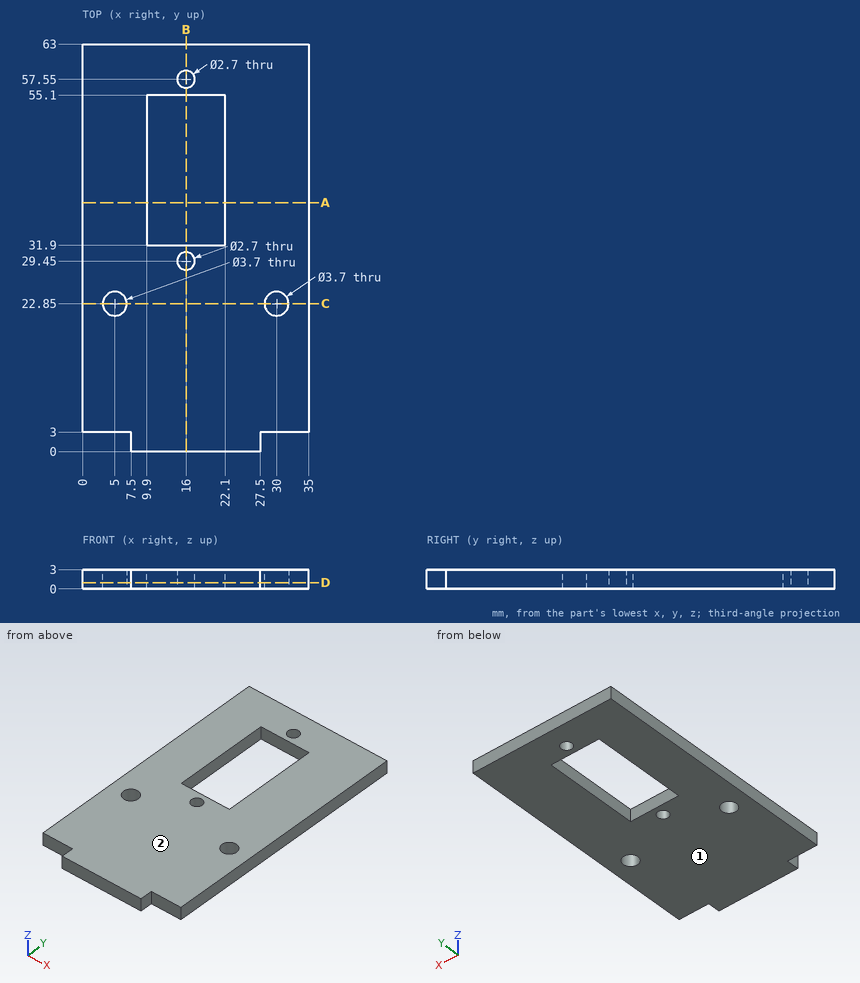
Here's the drawing with two shaded views (mm, measured from the low corner). I have some questions. Give positions to 0.01 mm unless a question says otherwise; leave off trailing zeros. Loops run counter-clockwise (first coordinate to the right, second up) from the corner with the lowest first, then second, coordinate; pieces in that order, holes last. Notation, with made-up numbers: M 14.25,0 L 35.25,0 A12 ccw 35.25,9 Z; hole C 5.5,40.25 d10. An arc over 180 degrees is marked long. One line per item, written item: value.
(1) Will these pins go through, and if not, where does the flat tip stop? pin 1 (0.9 mm diameter, centred on x = 5.5, z = 2, fed in from -Y); pin 2 (2 mm diameter, centred on x = 30, y = 22.85, fed in from +Z); pin 3 (5 mm diameter, centred on x = 5, y = 22.85, fed in from -Z).
Returned:
pin 1: y = 3
pin 2: through
pin 3: z = 0
(2) Suppose I cut it at D-D on z = 1. List the corners of the cut face in (x, y) for me.
Returned:
outline: M 0,3 L 7.5,3 L 7.5,0 L 27.5,0 L 27.5,3 L 35,3 L 35,63 L 0,63 Z; hole C 5,22.85 d3.7; hole M 9.9,31.9 L 22.1,31.9 L 22.1,55.1 L 9.9,55.1 Z; hole C 16,29.45 d2.7; hole C 16,57.55 d2.7; hole C 30,22.85 d3.7
(3) Suppose I cut it at C-C on y = 22.85. List the corners of the cut face in (x, z) for me.
Returned:
outline: M 0,0 L 3.15,0 L 3.15,3 L 0,3 Z; M 6.85,0 L 28.15,0 L 28.15,3 L 6.85,3 Z; M 31.85,0 L 35,0 L 35,3 L 31.85,3 Z
(4) I need wall thicknesses on line 1 (Y direction, x = 16, z = 2); line 2 (X direction, y = 36, z = 2.55); line 3 (Y direction, x = 14.5, z = 2.4). Which ranges of each line are inside material? Lowest first, please.
Returned:
line 1: 0 to 28.1, 30.8 to 31.9, 55.1 to 56.2, 58.9 to 63
line 2: 0 to 9.9, 22.1 to 35
line 3: 0 to 31.9, 55.1 to 63
(5) Suppose I cut it at A-A on y = 38.5. List the corners of the cut face in (x, z) for me.
Returned:
outline: M 0,0 L 9.9,0 L 9.9,3 L 0,3 Z; M 22.1,0 L 35,0 L 35,3 L 22.1,3 Z
(6) We'd pull the mould along Z, two halves only. Please class the marked faces 1 and 2: released by +Z, released by -Z, zero draft, split by the parting line, or undercut.
Returned:
face 1: released by -Z
face 2: released by +Z
(7) Suppose I cut it at B-B on x = 16. List the corners of the cut face in (y, z) for me, plus the area to 3 significant figures.
Returned:
outline: M 0,0 L 28.1,0 L 28.1,3 L 0,3 Z; M 30.8,0 L 31.9,0 L 31.9,3 L 30.8,3 Z; M 55.1,0 L 56.2,0 L 56.2,3 L 55.1,3 Z; M 58.9,0 L 63,0 L 63,3 L 58.9,3 Z
area: 103 mm^2
